Input: part model. Units: mm. Frame: model coordinates. A direction names the side the tool comes from. Coordinates: 2 decimals unless noted, no trailing zeros. Write each loop counter-clockwise with the first axis right and the second up, starting at its lowest first coordinate (ties: lowest second). Pieces come first, ordered by that corner, then holes.
1) Pin query (flat end, axial travel): pin 1 Ø5 at (x, y) = (1.5, -8.5) entering from +Z; pin 2 Ø6.5 at (x, z) = (-45, 0) entering from -Y; pin 3 Ø5 at (y, z) = (-6.5, 11.5) entering from -X. Return the tip coordinate at first contact, or that it passes through.
2) Section query C-C (y = -9.5). Output: boundary loops of the cut face in (x, z), then the cut area to 3 significant figures.
3) Set-up query: faces 4 (the cylindrical face through (50.076, -9.084, 15.77)), 5 (the cylindrical face through (-0.923, -1.479, 43.226)). Return all of +Z, -Z, +X, -X, +Y, -Y with unobstructed straight access to the full face (end or side cutting, diameter ignored); none if empty.
4) Line query: L1, parallel to Z at x = 0, y = -1.25; L2, parallel to X at y = -2.5, z = -14.5; L3, parallel to Y at x = -33, z = -33.5. Output: solid intervals per line, ascending.
5) Section query B-B (z = 0). Output: boundary loops of the cut face in (x, y).
6) Section query D-D (x = 26). Output: boundary loops of the cut face in (y, z), then the cut area to 3 significant figures.
7) Section query A-A (x = 0). Output: boundary loops of the cut face in (y, z), then the cut area to 3 significant figures.
8) Draft query along Z for faces 1 (the flat face through (28, 0, -28)), 2 (the cylindrical face through (62, -7.4, 19.52)), 3 (the flat face through (35, -3, 16)). Return one class per face: pulls with the +Z half, pulls with the -Z half, needs draft (parallel to the pull), parting line crosses it, or undercut.
from build123d import *

# Parameters (mm, degrees)
F0_R     = 65
F1_DEPTH = 15
F2_R     = 52.5
F3_DEPTH = 12
F5_D     = 4
F5_DEPTH = 25
F7_D     = 4
F7_DEPTH = 25
F8_R     = 37.5
F9_DEPTH = 25


with BuildPart() as f1:
    # F0 (on Front) → F1 (new body)
    with BuildSketch(Plane.XZ):
        Circle(F0_R)
    extrude(amount=F1_DEPTH)

    # F2 (on face) → F3 (cut)
    with BuildSketch(Plane.XZ.offset(15)):
        Circle(F2_R)
    extrude(amount=-F3_DEPTH, mode=Mode.SUBTRACT)

    # F5
    with Locations(Plane.XZ.offset(15)):
        with Locations((-58.75, 0), (0, 58.75), (58.75, 0), (0, -58.75)):
            Hole(F5_D / 2, depth=F5_DEPTH)

    # F7
    with Locations(Plane.XZ.offset(3)):
        with Locations((0, 45), (-45, 0), (45, 0), (0, -45)):
            Hole(F7_D / 2, depth=F7_DEPTH)

    # F8 (on face) → F9 (cut)
    with BuildSketch(Plane(origin=(0, 0, 0), x_dir=(-1, 0, 0), z_dir=(0, 1, 0))):
        Circle(F8_R)
    extrude(amount=-F9_DEPTH, mode=Mode.SUBTRACT)


solid = f1.part
Answer:
1. pin 1: stops at z = 65
1. pin 2: stops at y = -3
1. pin 3: stops at x = -64.37
2. outline: circle Ø130 at (0, 0); hole circle Ø4 at (-58.75, 0); hole circle Ø105 at (0, 0); hole circle Ø4 at (0, -58.75); hole circle Ø4 at (0, 58.75); hole circle Ø4 at (58.75, 0)
2. area: 4,560 mm2
3. face 4: -Y
3. face 5: +Y, -Y
4. L1: z = -65 to -60.75, -56.75 to -47, -43 to -37.5, 37.5 to 43, 47 to 56.75, 60.75 to 65
4. L2: x = -63.36 to -34.58, 34.58 to 63.36
4. L3: y = -3 to 0
5. outline: (-65, -15) - (-60.75, -15) - (-60.75, 0) - (-65, 0) - close; (-56.75, -15) - (-52.5, -15) - (-52.5, -3) - (-47, -3) - (-47, 0) - (-56.75, 0) - close; (-43, -3) - (-37.5, -3) - (-37.5, 0) - (-43, 0) - close; (37.5, -3) - (43, -3) - (43, 0) - (37.5, 0) - close; (47, -3) - (52.5, -3) - (52.5, -15) - (56.75, -15) - (56.75, 0) - (47, 0) - close; (60.75, -15) - (65, -15) - (65, 0) - (60.75, 0) - close
6. outline: (-15, -59.57) - (0, -59.57) - (0, -27.02) - (-3, -27.02) - (-3, -45.61) - (-15, -45.61) - close; (-15, 45.61) - (-3, 45.61) - (-3, 27.02) - (0, 27.02) - (0, 59.57) - (-15, 59.57) - close
6. area: 530 mm2
7. outline: (-15, -65) - (0, -65) - (0, -60.75) - (-15, -60.75) - close; (-15, -56.75) - (0, -56.75) - (0, -47) - (-3, -47) - (-3, -52.5) - (-15, -52.5) - close; (-15, 52.5) - (-3, 52.5) - (-3, 47) - (0, 47) - (0, 56.75) - (-15, 56.75) - close; (-15, 60.75) - (0, 60.75) - (0, 65) - (-15, 65) - close; (-3, -43) - (0, -43) - (0, -37.5) - (-3, -37.5) - close; (-3, 37.5) - (0, 37.5) - (0, 43) - (-3, 43) - close
7. area: 321 mm2
8. face 1: needs draft
8. face 2: parting line crosses it
8. face 3: undercut
